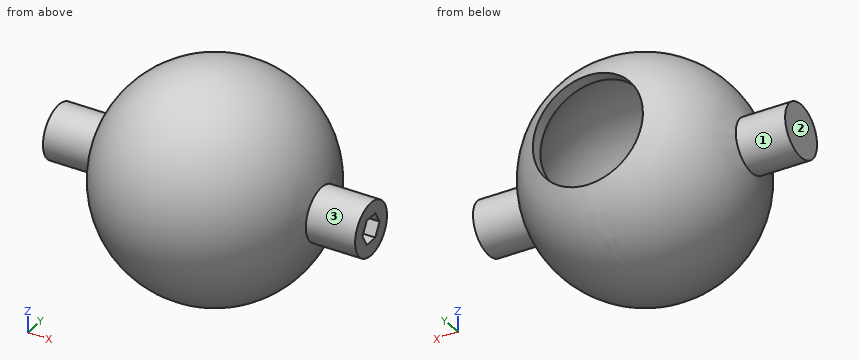
Autodesk Inventor part; units mm, degrees
ref_plane "Work Plane6" through (44, 0, 0) normal (1, 0, 0) x (0, 1, 0)
ref_plane "XZ Plane" through (0, 0, 0) normal (0, 1, 0) x (-1, 0, 0)
ref_plane "XY Plane" through (0, 0, 0) normal (0, 0, 1) x (1, 0, 0)
sketch "Sketch8" plane through (0, 0, 0) normal (1, 0, 0) x (0, 1, 0)
  arc A0 (0, -31.02) -> (0, 31.02) centre (0, 0) ccw
  line L0 (0, 31.02) -> (0, -31.02)
  line L1 (0, -49.5025) -> (0, 42.4391) construction
  dimension "radio" = 31.02
revolve "Revolution2" add sketch "Sketch8" angle 360 about axis through (0, 0, -49.5025) along (0, 0, 1)
sketch "Sketch15" plane through (0, 0, 0) normal (0, 1, 0) x (-1, 0, 0)
  circle A0 centre (0, 0) radius 15.51
  dimension "d35" = 31.02
extrude "Extrusion9" cut sketch "Sketch15" along normal up to surface
shell "Shell5" thickness 3 removed faces 2 at (0, 8.9547, 15.51) at (-6.3263, 0, 3.7266)
ref_plane "Work Plane6" through (44, 0, 0) normal (1, 0, 0) x (0, 1, 0)
sketch "Sketch13" plane through (44, 0, 0) normal (1, 0, 0) x (0, 1, 0)
  circle A0 centre (0, 0) radius 7.5
  dimension "d32" = 15
extrude "Extrusion8" add sketch "Sketch13" against normal up to next
mirror "Mirror1" about plane through (0, 0, 0) normal (1, 0, 0) of "Extrusion8"
sketch "Sketch16" plane through (44, 0, 0) normal (1, 0, 0) x (0, 0, -1)
  circle A0 centre (0, 0) radius 7.5
  circle A1 centre (0, 0) radius 4 construction
  line L0 (0, 4) -> (3.4641, 2)
  line L1 (3.4641, 2) -> (3.4641, -2)
  line L2 (3.4641, -2) -> (0, -4)
  line L3 (0, -4) -> (-3.4641, -2)
  line L4 (-3.4641, -2) -> (-3.4641, 2)
  line L5 (-3.4641, 2) -> (0, 4)
  dimension "d40" = 3.5
extrude "Extrusion10" cut sketch "Sketch16" against normal blind 10 contours L0 L1 L2 L3 L4 L5
equation "\"d35\" = radio"
properties part number "Dosificador" material "ABS Plastic"
Design review of the part built by this model. Coordinates are the model's own, in mm. Face numbers are marked on the shaded views. A direction names the side the tool comes from. Give positions to 0.01 mm unless a question says otherwise; leave off trailing zeros. Order: outer loops, then holes, each group sorted by start corner. A loop starts at its lowest first (then second) coordinate and runs counter-clockwise, first axis right, second up. Notation, with made-up numbers: (6, -13) - (15, -13) arc R19 cw to (15, -9) - close; hole circle Ø1 at (64.25, -25). An arc over 180 degrees is marked (long way). Use a Markdown table: item, result. Add a question column.
(1) Add section B-B on z = -5. Give the boundary of the cut face in (x, y).
(2) Add section D-D on z = -21.5. Give the boundary of the cut face in (x, y), then the cut area to 3 significant figures.
(3) Machinability: for the marked faces 1, 2 and 3, which of the approach directions +Z, -Z, +X, -X, +Y, -Y give a long, thin tool a straight path to every point of the face, cutting with its end or side? Answer none if there is none.
(4) Wall thickness on probe 1 along Z at (x, y) = (-2.5, -16); probe 2 along X at (y, z) = (-18, -7.5); probe 3 along X at (y, z) = (26, 0): over which ranges is each line inside the solid? List them lowest first. Write a range as [from, to].
(5) Add section C-C on x = -7. Give the boundary of the cut face in (y, z).
(6) Add section A-A on y = 0. Give the boundary of the cut face in (x, z).
(7) Clearance check with flat-ended pins moving along their axes: P1, Ø5, axis at y = -15, z = -22, coming from the -X side; P2, Ø6, axis at x = -10.5, y = 5, coming from the +Z side; P3, Ø3, axis at x = 10, y = 16.5, coming from the -Z side. State where each tip first meets the part, or that it passes through.
Report:
| question | item | result |
|---|---|---|
| 1 | outline | (-44, -5.59) - (-30.1, -5.59) arc R30.61 ccw to (30.1, -5.59) - (44, -5.59) - (44, 5.59) - (30.1, 5.59) arc R30.61 ccw to (14.68, 26.86) - (14.68, 23.34) arc R27.57 cw (long way) to (-14.68, 23.34) - (-14.68, 26.86) arc R30.61 ccw to (-30.1, 5.59) - (-44, 5.59) - close |
| 2 | outline | circle Ø44.72 at (0, 0); hole circle Ø35.94 at (0, 0) |
| 2 | area | 556 mm² |
| 3 | face 1 | -X |
| 3 | face 2 | +Z, -Z, -X, +Y, -Y |
| 3 | face 3 | +X |
| 4 | probe 1 | z = [-26.46, -22.87], [22.87, 26.46] |
| 4 | probe 2 | x = [-24.12, -20.12], [20.12, 24.12] |
| 4 | probe 3 | x = [-16.92, -15.51], [15.51, 16.92] |
| 5 | outline | (23.34, -13.84) arc R27.13 cw (long way) to (23.34, 13.84) - (26.86, 13.84) arc R30.22 ccw (long way) to (26.86, -13.84) - close |
| 6 | outline | (-44, -7.5) - (-30.1, -7.5) arc R31.02 ccw to (30.1, -7.5) - (44, -7.5) - (44, -3.46) - (34, -3.46) - (34, 3.46) - (44, 3.46) - (44, 7.5) - (30.1, 7.5) arc R31.02 ccw to (-30.1, 7.5) - (-44, 7.5) - close; hole circle Ø56.04 at (0, 0) |
| 7 | P1 | stops at x = -19.5 |
| 7 | P2 | stops at z = 29.8 |
| 7 | P3 | stops at z = -25.41 |
